Source: three-view drawing plus pictorial views. Frame: mm from the lowest corner of the part. A direction names the side the tool comes from. Give positions to 0.01 mm unless a question says otherwise; leave off trailing zeros. Order: outer loops, then holes, each group sorted by start corner. A loop starts at its lowest first (then second) coordinate and runs counter-clockwise, first axis right, second up. Notation, with made-up numbers: (49.5, 6.25) - (86.5, 6.25) arc R28 ccw to (86.5, 41.25) - close; hole circle Ø4 at (-23, -39.75). An arc over 180 degrees is marked (long way). Use CSV: the item, a comma, the result in double quotes.
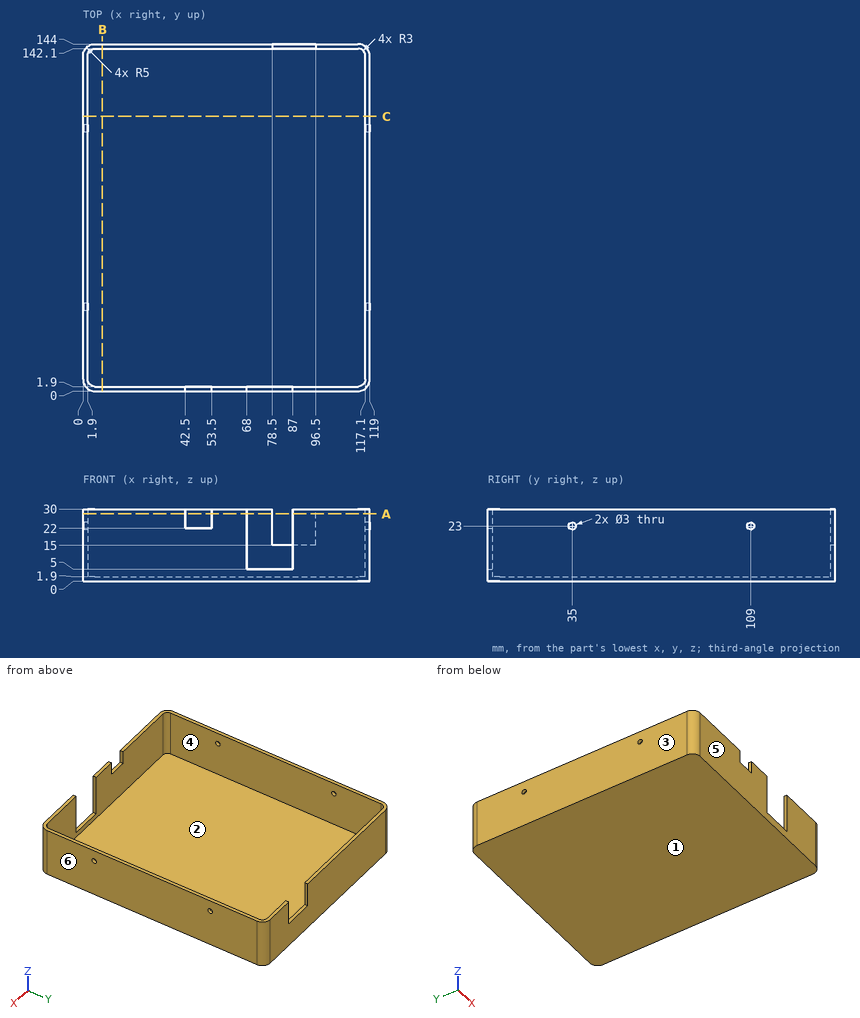
Item 1: Mould query, pull axis X, two halves, no side actions, for the marked faces 3, 4, 5 and 6. Classes: released by +X, released by -X, zero draft, split by the parting line, or undercut.
Filled in:
face 3,"released by -X"
face 4,"undercut"
face 5,"zero draft"
face 6,"released by +X"
Item 2: Set-up query: the marked faces 1 and 2. Return all of +Z, -Z, +X, -X, +Y, -Y with unobstructed straight access to the full face (end or side cutting, diameter ignored); none if empty.
Filled in:
face 1,"-Z, +X, -X, +Y, -Y"
face 2,"+Z"
Item 3: Section B-B on x = 8. Return the cut outline in (y, z).
Filled in:
outline,"(0, 0) - (144, 0) - (144, 30) - (142.1, 30) - (142.1, 1.9) - (1.9, 1.9) - (1.9, 30) - (0, 30) - close"
Item 4: Section A-A on z = 28. Return the cut outline in (x, y).
Filled in:
outline,"(0, 5) arc R5 ccw to (5, 0) - (42.5, 0) - (42.5, 1.9) - (4.9, 1.9) arc R3 cw to (1.9, 4.9) - (1.9, 139.1) arc R3 cw to (4.9, 142.1) - (78.5, 142.1) - (78.5, 144) - (5, 144) arc R5 ccw to (0, 139) - close; (53.5, 0) - (68, 0) - (68, 1.9) - (53.5, 1.9) - close; (87, 0) - (114, 0) arc R5 ccw to (119, 5) - (119, 139) arc R5 ccw to (114, 144) - (96.5, 144) - (96.5, 142.1) - (114.1, 142.1) arc R3 cw to (117.1, 139.1) - (117.1, 4.9) arc R3 cw to (114.1, 1.9) - (87, 1.9) - close"
Item 5: Material intervals for line 1 (X direction, y = 120, z = 15.25); line 2 (Y direction, x = 49.5, z = 7); line 3 (Z direction, x = 0.65, y = 35), sorted ascending. Write a range as from..to.
Filled in:
line 1,"x = 0..1.9, 117.1..119"
line 2,"y = 0..1.9, 142.1..144"
line 3,"z = 0..21.5, 24.5..30"
Item 6: First-contact query: pin 1 (5 mm diameter, centred on y = 109, z = 23, fed in from -X); pin 2 (1 mm diameter, centred on y = 0.5, z = 26, fed in from -X); pin 3 (0.6 mm diameter, centred on y = 143, z = 24, fed in from -X); pin 4 (1.5 mm diameter, centred on y = 1.5, z = 27, fed in from +X). Flat tips, straight axial feed; report the tip coordinate or a pass-through.
Filled in:
pin 1,"stops at x = 0"
pin 2,"stops at x = 2"
pin 3,"stops at x = 1.64"
pin 4,"stops at x = 118.18"
Item 7: Section C-C on y = 114. Return the cut outline in (x, z).
Filled in:
outline,"(0, 0) - (119, 0) - (119, 30) - (117.1, 30) - (117.1, 1.9) - (1.9, 1.9) - (1.9, 30) - (0, 30) - close"
